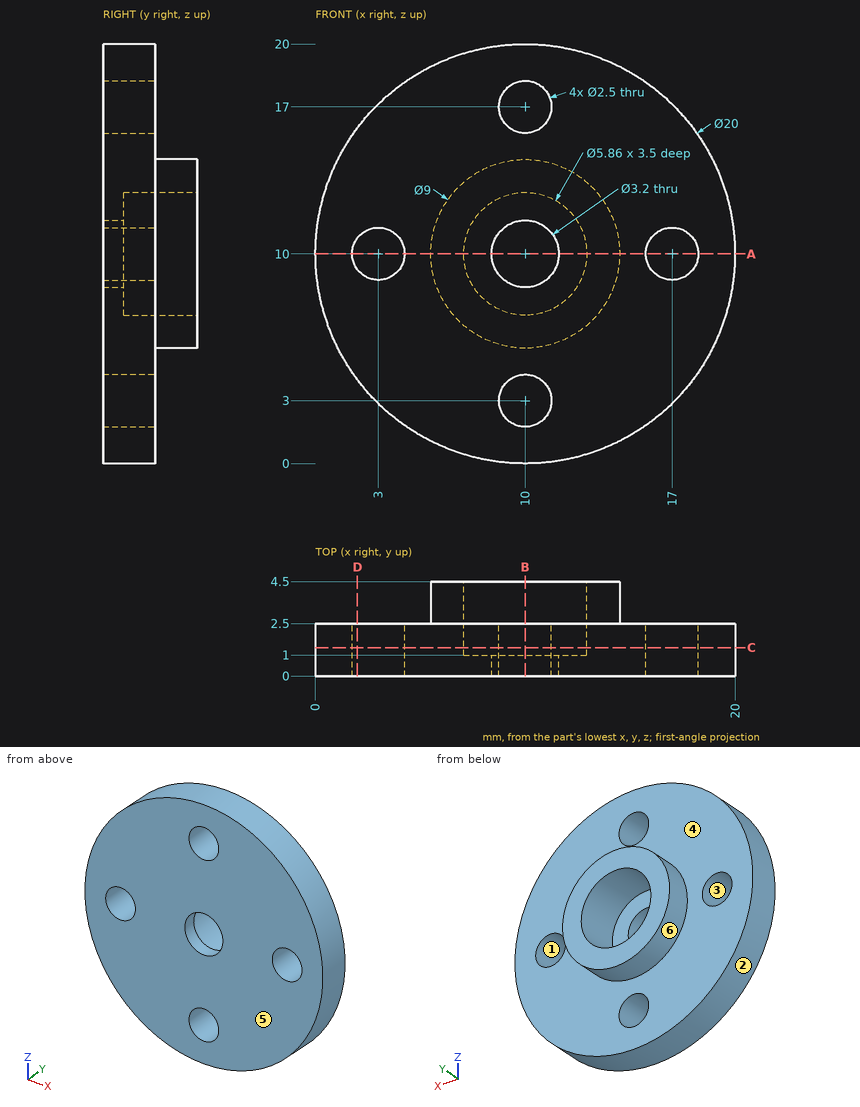
Answer from the drawing. Dimensions are ordinates in mm from the lowest x, y and z of the part. A direction names the side the tool comes from. Give positions to 0.01 mm unless a question says otherwise; leave off trailing zeros. Write each loop counter-clockwise with the first axis right and the second up, starting at its lowest first coordinate (ties: lowest second). Pieces come first, ordered by that corner, then holes. Notation, with made-up numbers: (70.25, 23) - (95.25, 23) arc R19 ccw to (95.25, 40) - close; hole circle Ø6 at (89, 13). An arc over 180 degrees is marked (long way). One line per item, written item: value. Start each with the question number.
1. Find section A-A (z = 10). Write down the section's boundary in (x, y).
2. Given pin 1 (5.5 mm diameter, centred on x = 10, z = 10, fed in from +Y); pin 2 (2 mm diameter, centred on x = 10, z = 3, fed in from +Y); pin 3 (3 mm diameter, centred on x = 17, z = 10, fed in from +Y), each flat-ended and moving along its own axis, determine where each tip first touches the part or whether it passes through.
3. For the marked faces 5 and 6, determine the directions among +Z, -Z, +X, -X, +Y, -Y from which every point of the face is accessible in a straight line to the end or side of a thin tool.
4. Find section D-D (x = 2). Write down the section's boundary in (y, z), then the cut area to 4 significant figures.
5. Find section B-B (x = 10). Write down the section's boundary in (y, z).
6. Find section C-C (y = 1.35). Write down the section's boundary in (x, z).
7. Consider probe 1 along X at (y, z) = (0.45, 10); probe 2 along Z at (x, y) = (10, 1.2). Determine where each line is inside the solid, lowest interval first.
8. For a pull along Z with two mould halves and no side action, classify the marked faces 1, 2, 3 and 4 as +Z half, -Z half, draft (parallel to the pull), parting line (faces both ways), or undercut.
Geometry results:
1. outline: (0, 0) - (1.75, 0) - (1.75, 2.5) - (0, 2.5) - close; (4.25, 0) - (8.4, 0) - (8.4, 1) - (7.07, 1) - (7.07, 4.5) - (5.5, 4.5) - (5.5, 2.5) - (4.25, 2.5) - close; (11.6, 0) - (15.75, 0) - (15.75, 2.5) - (14.5, 2.5) - (14.5, 4.5) - (12.93, 4.5) - (12.93, 1) - (11.6, 1) - close; (18.25, 0) - (20, 0) - (20, 2.5) - (18.25, 2.5) - close
2. pin 1: y = 1
2. pin 2: through
2. pin 3: y = 2.5
3. face 5: +Z, -Z, +X, -X, -Y
3. face 6: +Y
4. outline: (0, 4) - (2.5, 4) - (2.5, 9.25) - (0, 9.25) - close; (0, 10.75) - (2.5, 10.75) - (2.5, 16) - (0, 16) - close
4. area: 26.25 mm2
5. outline: (0, 0) - (2.5, 0) - (2.5, 1.75) - (0, 1.75) - close; (0, 4.25) - (2.5, 4.25) - (2.5, 5.5) - (4.5, 5.5) - (4.5, 7.07) - (1, 7.07) - (1, 8.4) - (0, 8.4) - close; (0, 11.6) - (1, 11.6) - (1, 12.93) - (4.5, 12.93) - (4.5, 14.5) - (2.5, 14.5) - (2.5, 15.75) - (0, 15.75) - close; (0, 18.25) - (2.5, 18.25) - (2.5, 20) - (0, 20) - close
6. outline: circle Ø20 at (10, 10); hole circle Ø2.5 at (3, 10); hole circle Ø5.86 at (10, 10); hole circle Ø2.5 at (10, 3); hole circle Ø2.5 at (10, 17); hole circle Ø2.5 at (17, 10)
7. probe 1: 0 to 1.75, 4.25 to 8.4, 11.6 to 15.75, 18.25 to 20
7. probe 2: 0 to 1.75, 4.25 to 7.07, 12.93 to 15.75, 18.25 to 20
8. face 1: undercut
8. face 2: parting line
8. face 3: undercut
8. face 4: draft
